CAD build for the part. Positions are in the model's coordinates, mm. Coordinates: 2 decimals unless noted, no trailing zeros. Loops run counter-clockwise (first coordinate to the right, second up) from the corner with the lowest first, then second, coordinate; pieces in that order, holes last. Notation, with made-up numbers: (13.25, 9) - (45.25, 9) arc R16 ccw to (45.25, 15) - close; hole circle Ø7 at (49.5, 10). An arc over 180 degrees is marked (long way). Put each result on its own line as item: value.
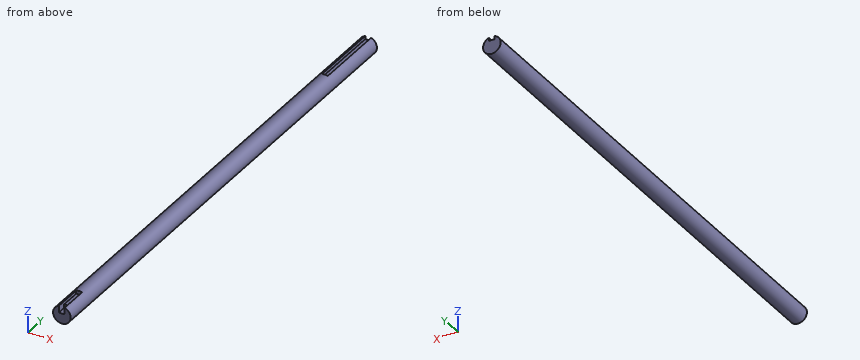
```python
from build123d import *

# Parameters (mm, degrees)
SKETCH1_R                = 6
BOSS_EXTRUDE1_DEPTH      = 254
BOSS_EXTRUDE1_DEPTH_BACK = 100
CUT_EXTRUDE3_START       = -100
SKETCH2_W                = 4
SKETCH2_H                = 5
CUT_EXTRUDE3_DEPTH       = 20
CUT_EXTRUDE3_DEPTH_BACK  = 0.0001
CUT_EXTRUDE4_START       = 254
SKETCH2_2_W              = 4
SKETCH2_2_H              = 5
CUT_EXTRUDE4_DEPTH       = 50
CUT_EXTRUDE6_START       = -100
SKETCH3_W                = 4
SKETCH3_H                = 10
CUT_EXTRUDE6_DEPTH       = 6


with BuildPart() as part:
    # Sketch1 → Boss-Extrude1 (new body, two sides)
    with BuildSketch(Plane(origin=(0, 0, 0), x_dir=(1, 0, 0), z_dir=(0, 1, 0))) as boss_extrude1_sk:
        Circle(SKETCH1_R)
    extrude(amount=BOSS_EXTRUDE1_DEPTH)
    extrude(boss_extrude1_sk.sketch, amount=-BOSS_EXTRUDE1_DEPTH_BACK)

    # Sketch2 → Cut-Extrude3 (cut, two sides)
    with BuildSketch(Plane(origin=(0, 0, 0), x_dir=(1, 0, 0), z_dir=(0, 1, 0)).offset(CUT_EXTRUDE3_START)) as cut_extrude3_sk:
        with Locations((0, -6)):
            Rectangle(SKETCH2_W, SKETCH2_H)
    extrude(amount=CUT_EXTRUDE3_DEPTH, mode=Mode.SUBTRACT)
    extrude(cut_extrude3_sk.sketch, amount=-CUT_EXTRUDE3_DEPTH_BACK, mode=Mode.SUBTRACT)

    # Sketch2<2> → Cut-Extrude4 (cut)
    with BuildSketch(Plane(origin=(0, 0, 0), x_dir=(1, 0, 0), z_dir=(0, 1, 0)).offset(CUT_EXTRUDE4_START)):
        with Locations((0, -6)):
            Rectangle(SKETCH2_2_W, SKETCH2_2_H)
    extrude(amount=-CUT_EXTRUDE4_DEPTH, mode=Mode.SUBTRACT)

    # Sketch3 → Cut-Extrude6 (cut)
    with BuildSketch(Plane(origin=(0, 0, 0), x_dir=(1, 0, 0), z_dir=(0, 1, 0)).offset(CUT_EXTRUDE6_START)):
        with Locations((0, -6)):
            Rectangle(SKETCH3_W, SKETCH3_H)
    extrude(amount=CUT_EXTRUDE6_DEPTH, mode=Mode.SUBTRACT)


solid = part.part
```
Q1. Slice it at D-D, the plane y = 211.5. Give the cut face in (x, z), then the cut area to 3 significant figures.
Determined:
outline: (-2, 3.5) - (-2, 5.66) arc R6 ccw (long way) to (2, 5.66) - (2, 3.5) - close
area: 104 mm2
Q2. Slice it at A-A, the plane x = 0. Give the cut face in (y, z), then the cut area to 3 significant figures.
Determined:
outline: (-100, -6) - (254, -6) - (254, 3.5) - (204, 3.5) - (204, 6) - (-80, 6) - (-80, 3.5) - (-94, 3.5) - (-94, 1) - (-100, 1) - close
area: 4,060 mm2
Q3. Wall check: L1, parallel to X at y = 223, z = -0.25; L2, parallel to Z at x = -5, y = -36.5. Give the ranges that are in metal, low to high. Write a range as from..to.
Determined:
L1: -5.99..5.99
L2: -3.32..3.32
Q4. Pin check, flat tips, straight feed: pin 1 Ø5 at (x, y) = (-4, 165) entering from -Z; pin 2 Ø1.2 at (x, y) = (0, 233.5) entering from +Z; pin 3 Ø1.5 at (x, y) = (-3.5, 206) entering from -Z. Stop position of each tip, or through.
Determined:
pin 1: z = -5.81
pin 2: z = 3.5
pin 3: z = -5.33
Q5. Slice it at C-C, the plane z = -2. Give the cut face in (x, y), then the cut area to 3 significant figures.
Determined:
outline: (-5.66, -100) - (5.66, -100) - (5.66, 254) - (-5.66, 254) - close
area: 4,010 mm2
Q6. Slice it at B-B, the plane y = -71. Give the cut face in (x, z), then the cut area to 3 significant figures.
Determined:
outline: circle Ø12 at (0, 0)
area: 113 mm2
